Autodesk Inventor part; units mm, degrees
ref_plane "Work Plane1" through (0, -15, 0) normal (1, 0, 0) x (0, 0, 1)
ref_plane "YZ Plane" through (0, 0, 0) normal (1, 0, 0) x (0, 1, 0)
ref_plane "XZ Plane" through (0, 0, 0) normal (0, 1, 0) x (-1, 0, 0)
sketch "Эскиз1" plane through (0, 0, 0) normal (0, 0, 1) x (1, 0, 0)
  line L0 (-6, 0) -> (6, 0) construction
  arc A0 (0.625, -29.2363) -> (-0.625, -29.2363) centre (0, -15) ccw
  line L1 (0, 20.1894) -> (0, -80.5364)
  line L2 (-48.09, 0) -> (48.09, 0)
  line L3 (-0.625, -29.2363) -> (-0.625, -34.2363)
  line L4 (-0.625, -6.5402) -> (-0.625, -13.29) construction
  line L5 (-2.7947, 3.5) -> (3.6722, 3.5) construction
  arc A1 (6.4152, -30.541) -> (-6.4152, -30.541) centre (0, -14.125) ccw
  arc A2 (-2.8732, -34.0308) -> (-0.625, -34.2363) centre (0, -15) ccw
  arc A3 (-4.9126, -32.2142) -> (-2.8732, -34.0308) centre (-2.5, -31.5588) ccw
  arc A4 (-4.9126, -32.2142) -> (-6.4152, -30.541) centre (-7.3251, -32.8695) ccw
  line L6 (0.625, -29.2363) -> (0.625, -34.2363)
  line L7 (0.625, -6.5402) -> (0.625, -13.29) construction
  arc A5 (0.625, -34.2363) -> (2.8732, -34.0308) centre (0, -15) ccw
  arc A6 (2.8732, -34.0308) -> (4.9126, -32.2142) centre (2.5, -31.5588) ccw
  arc A7 (6.4152, -30.541) -> (4.9126, -32.2142) centre (7.3251, -32.8695) ccw
  circle A8 centre (-2.5, -31.5588) radius 1.25
  circle A9 centre (2.5, -31.5588) radius 1.25
  dimension "d0" = 28.5
  dimension "d1" = 5
  dimension "d6" = 0.625
  dimension "d7" = 3.5
  dimension "d8" = 0.875
  dimension "d9" = 2.5
  dimension "d10" = 2.5
  dimension "d11" = 1.875
  dimension "d12" = 2.5
  dimension "d13" = 2.5
  dimension "d14" = 15
extrude "Базовый элемент" add sketch "Эскиз1" along normal blind 1.2
ref_plane "Work Plane1" through (0, -15, 0) normal (1, 0, 0) x (0, 0, 1)
equation "\"d0\" = ND"
equation "\"d1\" = SRB2"
equation "\"d6\" = 0.25 * SD5"
equation "\"d7\" = SRB1"
equation "\"d8\" = 0.25 * SRB1"
equation "\"d9\" = SD5"
equation "\"d10\" = SD5"
equation "\"d11\" = 0.75 * SD5"
equation "\"d12\" = SD5"
equation "\"d13\" = SD5"
equation "\"d14\" = 0.5 * WD"
equation "\"d2\" = SD"
equation "\"SD\" = 1.2"
equation "\"SRB1\" = 3.5"
equation "\"ND\" = 28.5"
equation "\"SRB2\" = 5"
equation "\"SD5\" = 2.5"
equation "\"SD3\" = 27.8"
equation "\"WDMAX\" = 32"
equation "\"SNB\" = 1.4"
equation "\"BUBRMI\" = 2.7"
properties part number "Кольцо A30 ГОСТ 13942-86" material "Сталь, мягкая"
CAD build for the part. Positions are in the model's coordinates, mm. A direction names the side the tool comes from. Coordinates: 2 decimals unless noted, no trailing zeros. Loops run counter-clockwise (first coordinate to the right, second up) from the corner with the lowest first, then second, coordinate; pieces in that order, holes last. Notation, with made-up numbers: (-24, 77) - (26, 77) arc R10 ccw to (26, 84) - close; hole circle Ø11 at (-37.75, 15.5). An arc over 180 degrees is marked (long way). Return JSON: item names as keys, results as strings.
1. Band-saw the part on B-B (y = -5). Give the cut face in (x, z), and give its area (3 significant figures).
Result:
{"outline": "(-15.08, 0) - (-10.15, 0) - (-10.15, 1.2) - (-15.08, 1.2) - close; (10.15, 0) - (15.08, 0) - (15.08, 1.2) - (10.15, 1.2) - close", "area": "11.8 mm2"}
2. Band-saw the part on A-A (x = -10.5). Give the cut face in (y, z).
Result:
{"outline": "(-28.28, 0) - (-24.63, 0) - (-24.63, 1.2) - (-28.28, 1.2) - close; (-5.37, 0) - (0.03, 0) - (0.03, 1.2) - (-5.37, 1.2) - close"}
3. 3-axis set-ups, long thin cutter, end or side, ignore diameter. For faces 1 (the cylindrical face through (3.172, -32.613, 0.592)), 2 (the flat face through (0.625, -32, 1)): which of +Z, -Z, +X, -X, +Y, -Y reach the whole face in a straight line?
Result:
{"face 1": "+Z, -Z", "face 2": "+Z, -Z, -Y"}
4. Drop a flat-ended pin along its axis: pin 1 (0.6 mm diameter, centred on y = -32.5, z = 0.5, fed in from -X). Give the stop position or say it passes through.
Result:
{"pin 1": "stops at x = -4.92"}
5. Probe L1, parallel to X at y = -32, z = 0.9 (3 decimals); L2, parallel to Y at x = -2.5, z = 0.3; L3, parallel to Y at x = 7, z = 0.15. List the from-to ranges inside material, lowest first. Write a range as from..to.
Result:
{"L1": "x = -4.981..-3.67, -1.33..-0.625, 0.625..1.33, 3.67..4.981", "L2": "y = -34.08..-32.81, -30.31..-29.03, -0.97..3.32", "L3": "y = -30.3..-27.41, -2.59..2.05"}
6. Band-saw the part on D-D (x = 0). Give the cut face in (y, z), and give its area (3 significant figures).
Result:
{"outline": "(-0.75, 0) - (3.5, 0) - (3.5, 1.2) - (-0.75, 1.2) - close", "area": "5.10 mm2"}
7. Mould opens along X. For faces 3 (the flat face through (-0.625, -32, 1)), 4 (the cylindrical face through (-1.736, -34.168, 0.592)), 5 (the cylindrical face through (-0.683, 3.487, 0.592)), 6 (the cylindrical face through (5.454, -31.211, 0.592)) say: released by +X, released by -X, zero draft, split by the parting line, or undercut.
Result:
{"face 3": "undercut", "face 4": "released by -X", "face 5": "split by the parting line", "face 6": "released by +X"}
8. Band-saw the part on C-C (z = 0.3). Give the cut face in (x, y) (3 decimals).
Result:
{"outline": "(-6.415, -30.541) arc R2.5 cw to (-4.913, -32.214) arc R2.5 ccw to (-2.873, -34.031) arc R19.241 ccw to (-0.625, -34.236) - (-0.625, -29.236) arc R14.25 cw (long way) to (0.625, -29.236) - (0.625, -34.236) arc R19.252 ccw to (2.873, -34.031) arc R2.5 ccw to (4.913, -32.214) arc R2.5 cw to (6.415, -30.541) arc R17.625 ccw (long way) to start; hole circle Ø2.5 at (-2.5, -31.559); hole circle Ø2.5 at (2.5, -31.559)"}
